```python
from build123d import *

# Parameters (mm, degrees)
SKETCH1_W           = 200
SKETCH1_H           = 90
SKETCH1_R           = 1.5
BOSS_EXTRUDE1_DEPTH = 5
SKETCH2_W           = 140
SKETCH2_H           = 90
CUT_EXTRUDE1_DEPTH  = 142.850408897
SKETCH3_R           = 1.5
CUT_EXTRUDE2_DEPTH  = 137.124210251
SKETCH4_W           = 90
SKETCH4_H           = 5
BOSS_EXTRUDE2_DEPTH = 100


with BuildPart() as part:
    # Sketch1 → Boss-Extrude1 (new body)
    with BuildSketch(Plane(origin=(0, 0, 0), x_dir=(1, 0, 0), z_dir=(0, 1, 0))):
        with Locations((3.97934472, -51.35784543)):
            Rectangle(SKETCH1_W, SKETCH1_H)
        with Locations(Location((-86.02065528, -9.35784543, 0), (0, 0, 270))):
            Circle(SKETCH1_R, mode=Mode.SUBTRACT)
        with Locations(Location((-86.02065528, -93.35784543, 0), (0, 0, 270))):
            Circle(SKETCH1_R, mode=Mode.SUBTRACT)
        with Locations(Location((93.97934472, -9.35784543, 0), (0, 0, 270))):
            Circle(SKETCH1_R, mode=Mode.SUBTRACT)
        with Locations(Location((93.97934472, -93.35784543, 0), (0, 0, 270))):
            Circle(SKETCH1_R, mode=Mode.SUBTRACT)
    extrude(amount=BOSS_EXTRUDE1_DEPTH)

    # Sketch2 → Cut-Extrude1 (cut, through all)
    with BuildSketch(Plane(origin=(0, 5, 0), x_dir=(1, 0, 0), z_dir=(0, 1, 0))):
        with Locations((33.97934472, -51.35784543)):
            Rectangle(SKETCH2_W, SKETCH2_H)
    extrude(amount=-CUT_EXTRUDE1_DEPTH, mode=Mode.SUBTRACT)

    # Sketch3 → Cut-Extrude2 (cut, through all)
    with BuildSketch(Plane(origin=(0, 5, 0), x_dir=(1, 0, 0), z_dir=(0, 1, 0))):
        with Locations(Location((-46.006691674, -13.85784543, 0), (0, 0, 270))):
            Circle(SKETCH3_R)
        with Locations(Location((-46.006691674, -89.85784543, 0), (0, 0, 270))):
            Circle(SKETCH3_R)
    extrude(amount=-CUT_EXTRUDE2_DEPTH, mode=Mode.SUBTRACT)

    # Sketch4 → Boss-Extrude2 (add)
    with BuildSketch(Plane(origin=(-36.02065528, 0, 0), x_dir=(0, 0, -1), z_dir=(1, 0, 0))):
        with Locations((-51.35784543, 2.5)):
            Rectangle(SKETCH4_W, SKETCH4_H)
    extrude(amount=BOSS_EXTRUDE2_DEPTH)


solid = part.part
```
The model under review builds one solid part; all positions refer to its coordinate system, in mm. Round coordinates to 2 decimals unless told otherwise and drop trailing zeros. Answer as a JSON object with one key per item and string values. Group by question number.
1) Mouldability with a two-part tool opening along Z and no side actions: class faces 1 (the face through (-17, 2, 6.358)), 2 (the face through (-17, 2, 96.358)), 3 (the face through (-84.533, 2.465, 9.163)), 4 (the face through (-17, 0, 52)) as released by +Z, released by -Z, zero draft, split by the parting line, or undercut.
2) For line 1 (X direction, y = 1.6, z = 13); line 2 (X direction, y = 2.85, z = 92.5), list the stretches that pass through material, from the lowest coordinate up. Write a range as [from, to].
3) For pin 1 Ø2.5 at (x, z) = (-46.01, 89.86) entering from +Y, flat-tipped, find the tip position at first contact; note if it passes through.
Result set:
{
 "1": {"face 1": "released by -Z", "face 2": "released by +Z", "face 3": "undercut", "face 4": "zero draft"},
 "2": {"line 1": "[-96.02, -47.24], [-44.78, 63.98]", "line 2": "[-96.02, -87.25], [-84.79, 63.98]"},
 "3": {"pin 1": "through"}
}
